```python
from build123d import *

# Parameters (mm, degrees)
SKETCH005_W     = 7.4
SKETCH005_H     = 10.4
SKETCH005_R     = 1.58
PAD003_DEPTH    = 0.985
PAD001_DEPTH    = 4
POCKET_DEPTH    = 1.35
SKETCH004_R     = 1.6
POCKET001_DEPTH = 3.251
SKETCH006_R     = 2
POCKET002_DEPTH = 0.02
PAD_DEPTH       = 0.2625


with BuildPart() as pad003:
    # Sketch005 → Pad003 (new body, symmetric)
    with BuildSketch(Plane.XZ.offset(-1)):
        with Locations((2.54, 8.4)):
            Rectangle(SKETCH005_W, SKETCH005_H)
        with Locations((2.54, 10.2)):
            Circle(SKETCH005_R, mode=Mode.SUBTRACT)
    extrude(amount=PAD003_DEPTH, both=True)


with BuildPart() as pocket002:
    # Sketch001 → Pad001 (new body, symmetric)
    with BuildSketch(Plane.YZ.offset(2.54)):
        Polygon((0, 3), (-1.25, 3), (-1.25, 13.99), (-1.24, 14), (2, 14), (2, 3), align=None)
    extrude(amount=PAD001_DEPTH, both=True)

    # Sketch003 → Pocket (cut)
    with BuildSketch(Plane(origin=(2.54, -1.25, 0), x_dir=(0, 0, -1), z_dir=(0, -1, 0))):
        with BuildLine():
            Line((-12.219868, 0.5), (-12.219868, -0.5))
            Line((-12.219868, -0.5), (-11.719868, -0.5))
            ThreePointArc((-11.719868, -0.5), (-11, -1.385641), (-9.873078, -1.566245))
            Line((-9.623078, -1.999257), (-9.873078, -1.566245))
            Line((-8.757053, -1.499257), (-9.623078, -1.999257))
            Line((-9.007053, -1.066245), (-8.757053, -1.499257))
            ThreePointArc((-9.007053, -1.066245), (-8.6, 0), (-9.007053, 1.066245))
            Line((-8.757053, 1.499257), (-9.007053, 1.066245))
            Line((-9.623078, 1.999257), (-8.757053, 1.499257))
            Line((-9.873078, 1.566245), (-9.623078, 1.999257))
            ThreePointArc((-9.873078, 1.566245), (-11, 1.385641), (-11.719868, 0.5))
            Line((-12.219868, 0.5), (-11.719868, 0.5))
        make_face()
    extrude(amount=-POCKET_DEPTH, mode=Mode.SUBTRACT)

    # Sketch004 → Pocket001 (cut, through all)
    with BuildSketch(Plane(origin=(2.54, -1.25, 0), x_dir=(0, 0, -1), z_dir=(0, -1, 0))):
        with Locations((-10.2, 0)):
            Circle(SKETCH004_R)
    extrude(amount=-POCKET001_DEPTH, mode=Mode.SUBTRACT)

    # Sketch006 → Pocket002 (cut)
    with BuildSketch(Plane(origin=(2.54, 2, 0), x_dir=(0, 0, 1), z_dir=(0, 1, 0))):
        with BuildLine():
            Line((5.8, 3), (12.2, 3))
            ThreePointArc((13, 2.2), (12.765685, 2.765685), (12.2, 3))
            Line((13, 2.2), (13, -2.2))
            ThreePointArc((12.2, -3), (12.765685, -2.765685), (13, -2.2))
            Line((12.2, -3), (5.8, -3))
            ThreePointArc((5, -2.2), (5.234315, -2.765685), (5.8, -3))
            Line((5, -2.2), (5, 2.2))
            ThreePointArc((5.8, 3), (5.234315, 2.765685), (5, 2.2))
        make_face()
        with Locations((10.2, 0)):
            Circle(SKETCH006_R, mode=Mode.SUBTRACT)
    extrude(amount=-POCKET002_DEPTH, mode=Mode.SUBTRACT)


with BuildPart() as to_126_3_vertical:
    # Sketch → Pad (new body, symmetric)
    with BuildSketch(Plane.XZ):
        Polygon((-0.4, 0.3025), (-0.4, 0), (-0.4, -9.679469), (0, -9.75), (0.4, -9.679469), (0.4, 0), (0.4, 0.3025), (0.4, 3.73), (-0.4, 3.73), align=None)
        Polygon((1.81, 0.33), (2.14, 0), (2.14, -9.679469), (2.54, -9.75), (2.94, -9.679469), (2.94, 0), (3.27, 0.33), (3.27, 3.73), (1.81, 3.73), align=None)
        Polygon((4.68, 0.3025), (4.68, 0), (4.68, -9.679469), (5.08, -9.75), (5.48, -9.679469), (5.48, 0), (5.48, 0.3025), (5.48, 3.73), (4.68, 3.73), align=None)
    extrude(amount=PAD_DEPTH, both=True)

    add(pad003.part)
    add(pocket002.part)


solid = to_126_3_vertical.part
```
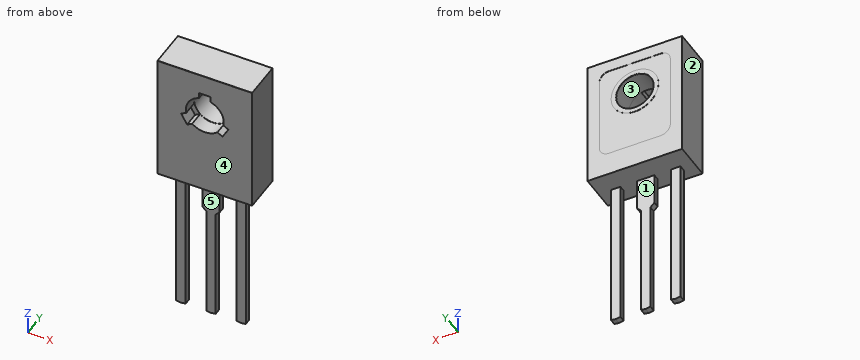
Geometry: final body of the model. Coordinates: model frame, mm. Face numbers are marked on the shaded views. A direction names the side the tool comes from. Coordinates: 2 decimals unless noted, no trailing zeros. Write each loop counter-clockwise with the first axis right and the second up, starting at its lowest first coordinate (ties: lowest second). Pieces come first, ordered by that corner, then holes. Notation, with made-up numbers: M 89,-9 L 135,-9 A19 cw 135,11 Z; hole C 83.5,-3.5 d4. An arc over 180 degrees is marked long. Use CSV: the item, a comma, the result in double quotes. Start each with the question number.
1. Reachability of the marked faces 4 and 5 from +Z, -Z, +X, -X, +Y, -Y: full face, straight path, thin tool, end or side. Return the list, or none.
2. Cut plane B-B on z = 10.2. Return the cut outline in (x, y) (3 decimals), plus the area to 3 significant figures.
3. First-contact query: P1, Ø0.6, axis at y = 0, z = -4.5, coming from the -X side; P2, Ø1.6, axis at x = 2.5, z = -5, coming from the +Y side. Flat tips, straight axial feed; report the tip coordinate or a pass-through.
4. Cut plane C-C on y = 1.55. Return the cut outline in (x, z).
5. Cut plane A-A on z = -0.5. Return the cut outline in (x, y), plus the area to 3 significant figures.
6. Mould query, pull axis X, two halves, no side actions, for the marked faces 1, 2 and 3. Classes: pulls with the +X half, pulls with the -X half, needs draft (parallel to the pull), parting line crosses it, or undercut.
7. Ray query, probe 1 along X at (y, z) = (0.05, -3.5); probe 2 along Z at (x, y) = (2.54, 0.7); probe 3 along X at (y, z) = (1.25, 10). Return the intervals inside material, ascending.
Entries:
1,face 4,"+Z, -Z, +X, -X, -Y"
1,face 5,"-Z, +X, -X, -Y"
2,outline,"M -1.46,-1.25 L 0.94,-1.25 L 0.94,0.015 L 0.96,0.015 L 0.96,1.985 L 0.94,1.985 L 0.94,2 L 0.54,2 L 0.54,1.985 L -0.46,1.985 L -0.46,2 L -1.46,2 Z; M 4.12,0.015 L 4.14,0.015 L 4.14,-1.25 L 6.54,-1.25 L 6.54,2 L 5.54,2 L 5.54,1.985 L 4.54,1.985 L 4.54,2 L 4.14,2 L 4.14,1.985 L 4.12,1.985 Z"
2,area,"15.6 mm²"
3,P1,"x = -0.4"
3,P2,"y = 0.26"
4,outline,"M -1.46,3 L 6.54,3 L 6.54,14 L -1.46,14 Z; hole C 2.54,10.2 d3.16"
5,outline,"M -0.4,-0.26 L 0.4,-0.26 L 0.4,0.26 L -0.4,0.26 Z; M 2.14,-0.26 L 2.94,-0.26 L 2.94,0.26 L 2.14,0.26 Z; M 4.68,-0.26 L 5.48,-0.26 L 5.48,0.26 L 4.68,0.26 Z"
5,area,"1.26 mm²"
6,face 1,"needs draft"
6,face 2,"pulls with the -X half"
6,face 3,"undercut"
7,probe 1,"-0.4 to 0.4, 2.14 to 2.94, 4.68 to 5.48"
7,probe 2,"3 to 8.62, 11.78 to 14"
7,probe 3,"-1.46 to 0.97, 4.11 to 6.54"
